Source: CAD feature listing. Evaluate the final solid. Frame: model axes, mm. Face numbers are marked on the shaded views. A direction names the side the tool comes from. Coordinates: 2 decimals unless noted, no trailing zeros. Loops run counter-clockwise (first coordinate to the right, second up) from the corner with the lowest first, then second, coordinate; pieces in that order, holes last. Notation, with made-up numbers: (60.5, 71.25) -> (90.5, 71.25) arc R26 cw to (90.5, 104.25) -> close; hole circle Ø2 at (83, 36). An arc over 180 degrees is marked (long way). Answer as a JSON object with one key per item and string values. Group by question number.
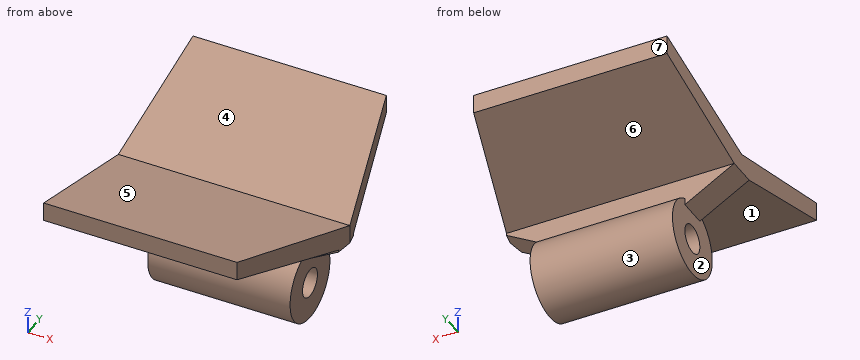
from build123d import *

# Parameters (mm, degrees)
F0_R     = 4
F0_R_2   = 1.5
F1_DEPTH = 15
F3_DEPTH = 1.5
F5_DEPTH = 24.3923048454
F7_DEPTH = 25


with BuildPart() as f1:
    # F0 (on Right) → F1 (new body)
    with BuildSketch(Plane.YZ):
        Circle(F0_R)
        Circle(F0_R_2, mode=Mode.SUBTRACT)
    extrude(amount=F1_DEPTH)

    # F2 (on Front) → F3 (join, symmetric)
    with BuildSketch(Plane.XZ):
        Polygon((-5.1961524227, 6), (0, 3), (14, 3), (19.1961524227, 6), (19.1961524227, 8), (-5.1961524227, 8), align=None)
    extrude(amount=F3_DEPTH, both=True)

    # F4 (on face) → F5 (join, through all)
    with BuildSketch(Plane(origin=(-5.1961524227, 0, 0), x_dir=(0, -1, 0), z_dir=(-1, 0, 0))):
        Polygon((15, 12.0192378865), (0, 8), (1.5, 6), (15, 10.0192378865), align=None)
        Polygon((-1.5, 6), (0, 8), (-15, 12.0192378865), (-15, 10.0192378865), align=None)
    extrude(amount=-F5_DEPTH)

    # F6 (on Top) → F7 (cut)
    with BuildSketch(Plane.XY):
        Polygon((14.137943439, 18.8774929223), (19.1961524227, 0), (14.137943439, -18.8774929223), (27.2481460124, -18.8774929223), (27.2481460124, 0), (27.2481460124, 18.8774929223), align=None)
    extrude(amount=F7_DEPTH, mode=Mode.SUBTRACT)


solid = f1.part
1. Reachability of the marked faces 5, 6 and 7 from +Z, -Z, +X, -X, +Y, -Y: full face, straight path, thin tool, end or side. Return the list, or none.
2. Section query C-C on z = 7.5. Return loops of the section in (x, y).
3. Pin query (flat end, axial travel): pin 1 Ø8 at (x, z) = (6.5, 2.5) entering from -Y; pin 2 Ø5 at (x, y) = (1, -1.5) entering from +Z; pin 3 Ø8 at (y, z) = (8.5, -2.5) entering from -X; pin 4 Ø8.5 at (y, z) = (-1.5, -2) entering from -X. Return the tip coordinate at first contact, or that it passes through.
4. Ray query, L1, parallel to Z at x = 9.5, y = 0; L2, parallel to Y at x = 17, z = 5; L3, parallel to X at y = 2.5, z = -1. Return the intervals inside material, ascending.
5. Section query A-A on x = 4.5. Return loops of the section in (y, z), then the cut area to 3 significant figures.
6. Section query B-B on z = 0. Return loops of the section in (x, y), then the cut area to 3 significant figures.
7. Section query D-D on x = 16.75. Return loops of the section in (y, z).
8. Mould query, pull axis Y, two halves, no side actions, for the marked faces 1, 2, 3 and 4. Classes: pulls with the +Y half, pulls with the -Y half, needs draft (parallel to the pull), parting line crosses it, or undercut.
Solved:
{
 "1": {"face 5": "+Z, +X, -X", "face 6": "+X, -X, +Y", "face 7": "+Z, -Z, +X, -X, +Y"},
 "2": {"outline": "(-5.2, -6.54) -> (17.44, -6.54) -> (19.2, 0) -> (17.44, 6.54) -> (-5.2, 6.54) -> close"},
 "3": {"pin 1": "y = -4", "pin 2": "z = 9.07", "pin 3": "through", "pin 4": "x = 0"},
 "4": {"L1": "-4 to -1.5, 1.5 to 8", "L2": "-1.5 to 1.5", "L3": "0 to 15"},
 "5": {"outline": "(-15, 10.02) -> (-1.5, 6) -> (-1.5, 3.71) arc R4 ccw (long way) to (1.5, 3.71) -> (1.5, 6) -> (15, 10.02) -> (15, 12.02) -> (0, 8) -> (-15, 12.02) -> close; hole circle Ø3 at (0, 0)", "area": "116 mm^2"},
 "6": {"outline": "(0, -4) -> (15, -4) -> (15, -1.5) -> (0, -1.5) -> close; (0, 1.5) -> (15, 1.5) -> (15, 4) -> (0, 4) -> close", "area": "75.0 mm^2"},
 "7": {"outline": "(-9.13, 8.27) -> (-1.5, 6) -> (-1.5, 4.59) -> (1.5, 4.59) -> (1.5, 6) -> (9.13, 8.27) -> (9.13, 10.45) -> (0, 8) -> (-9.13, 10.45) -> close"},
 "8": {"face 1": "pulls with the -Y half", "face 2": "needs draft", "face 3": "parting line crosses it", "face 4": "undercut"}
}
